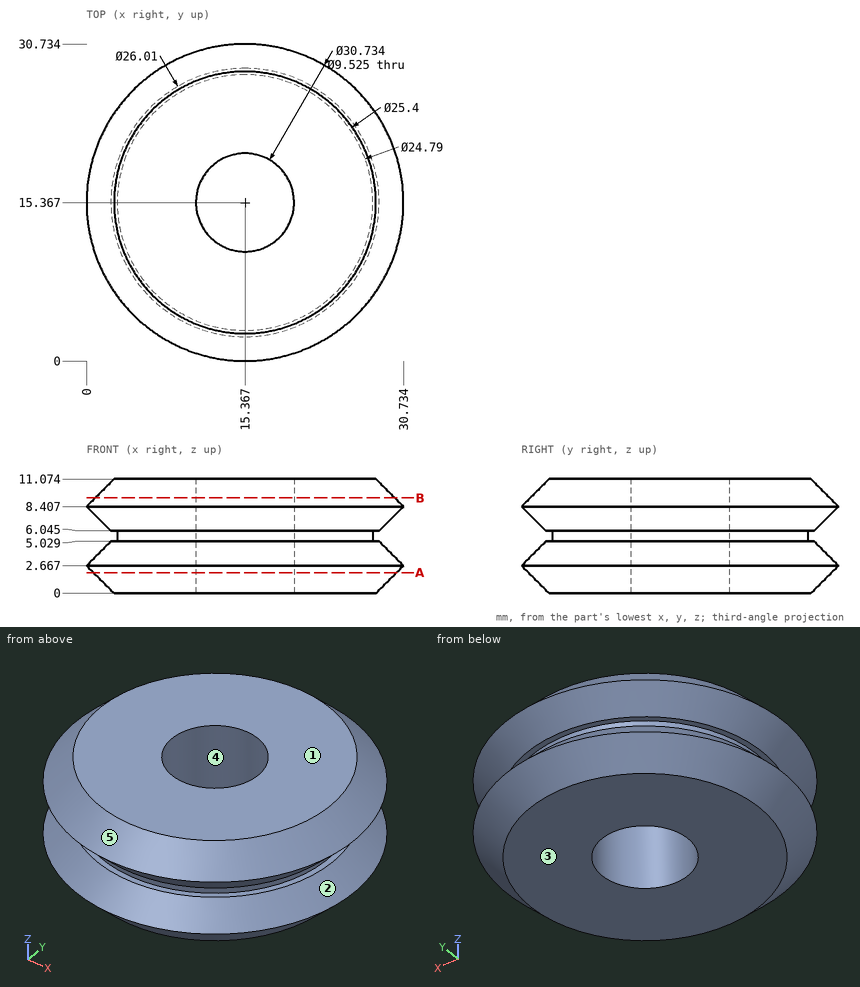
Source: three-view drawing plus pictorial views. Frame: mm from the lowest corner of the part. A direction names the side the tool comes from. Coordinates: 2 decimals unless noted, no trailing zeros. Loops run counter-clockwise (first coordinate to the right, second up) from the corner with the lowest first, then second, coordinate; pieces in that order, holes last. Notation, with made-up numbers: (6, -14) - (10, -14) arc R23 ccw to (10, 18) - close; hole circle Ø6 at (2.5, 2). An arc over 180 degrees is marked (long way). Answer in a Markdown table with one row per item. Add a question column.
Item 1: Section query A-A on z = 2. Return the cut outline in (x, y) (1 decimal).
Item 2: Mould query, pull axis X, two halves, no side actions, for the marked faces 3, 4 and 5. Classes: released by +X, released by -X, zero draft, split by the parting line, or undercut.
Item 3: Line query: line 1 along Z through (x, y) = (11, 27) (1 decimal); line 2 along X through (y, z) = (19, 7.25) (1 decimal); line 3 along X through (y, z) = (16, 1.75) (1 decimal). Output: solid intervals per line, ascending. Write a range as [from, to].
Item 4: Access query for the marked faces 1 and 2. Directions: +Z, -Z, +X, -X, +Y, -Y. A direction counts if a zero-diameter tool reaches every point of the face in a straight line with its end or side. Return the directions, or none.
Item 5: Contact query for flat-ended pins moving along their axis: P1, Ø6, axis at y = 26.5, z = 7, coming from the -X side (1 decimal); P2, Ø1.5, axis at x = 24, y = 4, coming from the +Z side; P3, Ø1.5, axis at y = 8, z = 5.5, coming from the -X side. Output: stop coordinate, or through.
Item 6: Section query B-B on z = 9.25. Return the cut outline in (x, y) (1 decimal).
Recorded:
| question | item | result |
|---|---|---|
| 1 | outline | circle Ø29.4 at (15.4, 15.4); hole circle Ø9.5 at (15.4, 15.4) |
| 2 | face 3 | zero draft |
| 2 | face 4 | undercut |
| 2 | face 5 | split by the parting line |
| 3 | line 1 | [0, 5], [6, 11.1] |
| 3 | line 2 | [1.6, 12.3], [18.4, 29.1] |
| 3 | line 3 | [0.9, 10.6], [20.1, 29.8] |
| 4 | face 1 | +Z, +X, -X, +Y, -Y |
| 4 | face 2 | none |
| 5 | P1 | x = 2.6 |
| 5 | P2 | z = 10.25 |
| 5 | P3 | x = 4.19 |
| 6 | outline | circle Ø29 at (15.4, 15.4); hole circle Ø9.5 at (15.4, 15.4) |
